```python
from build123d import *

# Parameters (mm, degrees)
SKETCH2_W           = 88.9
SKETCH2_H           = 152.4
BOSS_EXTRUDE1_DEPTH = 10.16
SKETCH5_W           = 57.15
SKETCH5_H           = 50.8
BOSS_EXTRUDE2_DEPTH = 133.35
SKETCH6_R           = 2.5
CUT_EXTRUDE1_DEPTH  = 11.16
SKETCH7_R           = 10.5
CUT_EXTRUDE2_DEPTH  = 58.15
SKETCH8_R           = 16.5
CUT_EXTRUDE3_DEPTH  = 54.15
SKETCH9_R           = 19.5
CUT_EXTRUDE4_DEPTH  = 16.51
BOSS_EXTRUDE3_DEPTH = 3
SKETCH12_R          = 9.525
CUT_EXTRUDE6_DEPTH  = 12.7


with BuildPart() as part:
    # Sketch2 → Boss-Extrude1 (new body)
    with BuildSketch(Plane(origin=(0, 0, 0), x_dir=(1, 0, 0), z_dir=(0, 1, 0))):
        with Locations((8.89, -19.614444444)):
            Rectangle(SKETCH2_W, SKETCH2_H)
    extrude(amount=BOSS_EXTRUDE1_DEPTH)

    # Sketch5 → Boss-Extrude2 (add)
    with BuildSketch(Plane(origin=(0, 10.16, 0), x_dir=(1, 0, 0), z_dir=(0, 1, 0))):
        with Locations((-6.985, -19.614444444)):
            Rectangle(SKETCH5_W, SKETCH5_H)
    extrude(amount=BOSS_EXTRUDE2_DEPTH)

    # Sketch6 → Cut-Extrude1 (cut, through all)
    with BuildSketch(Plane(origin=(0, 10.16, 0), x_dir=(1, 0, 0), z_dir=(0, 1, 0))):
        with Locations((35.84, -88.314444444)):
            Circle(SKETCH6_R)
        with Locations((45.84, -88.314444444)):
            Circle(SKETCH6_R)
        with Locations((-28.06, -88.314444444)):
            Circle(SKETCH6_R)
        with Locations((-18.06, -88.314444444)):
            Circle(SKETCH6_R)
        with Locations((-28.06, 49.085555556)):
            Circle(SKETCH6_R)
        with Locations((-18.06, 49.085555556)):
            Circle(SKETCH6_R)
        with Locations((35.84, 49.085555556)):
            Circle(SKETCH6_R)
        with Locations((45.84, 49.085555556)):
            Circle(SKETCH6_R)
    extrude(amount=-CUT_EXTRUDE1_DEPTH, mode=Mode.SUBTRACT)

    # Sketch7 → Cut-Extrude2 (cut, through all)
    with BuildSketch(Plane(origin=(21.59, 0, 0), x_dir=(0, 0, -1), z_dir=(1, 0, 0))):
        with Locations((-19.614444444, 119.38)):
            Circle(SKETCH7_R)
    extrude(amount=-CUT_EXTRUDE2_DEPTH, mode=Mode.SUBTRACT)

    # Sketch8 → Cut-Extrude3 (cut)
    with BuildSketch(Plane.ZY.offset(35.56)):
        with Locations((19.614444444, 119.38)):
            Circle(SKETCH8_R)
    extrude(amount=-CUT_EXTRUDE3_DEPTH, mode=Mode.SUBTRACT)

    # Sketch9 → Cut-Extrude4 (cut)
    with BuildSketch(Plane.ZY.offset(35.56)):
        with Locations((19.614444444, 119.38)):
            Circle(SKETCH9_R)
    extrude(amount=-CUT_EXTRUDE4_DEPTH, mode=Mode.SUBTRACT)

    # Sketch10 → Boss-Extrude3 (add)
    with BuildSketch(Plane(origin=(21.59, 0, 0), x_dir=(0, 0, -1), z_dir=(1, 0, 0))):
        with BuildLine():
            Line((-29.348407204, 123.317), (-29.348407204, 115.443))
            ThreePointArc((-29.348407204, 115.443), (-30.114444444, 119.38), (-29.348407204, 123.317))
        make_face()
        with BuildLine():
            Line((-9.880481685, 115.443), (-9.880481685, 123.317))
            ThreePointArc((-9.880481685, 123.317), (-9.114444444, 119.38), (-9.880481685, 115.443))
        make_face()
    extrude(amount=-BOSS_EXTRUDE3_DEPTH)

    # Sketch12 → Cut-Extrude6 (cut)
    with BuildSketch(Plane(origin=(0, 10.16, 0), x_dir=(1, 0, 0), z_dir=(0, 1, 0))):
        with Locations((53.34, -70.414444444)):
            Circle(SKETCH12_R)
        with Locations((53.34, 31.185555556)):
            Circle(SKETCH12_R)
    extrude(amount=-CUT_EXTRUDE6_DEPTH, mode=Mode.SUBTRACT)


solid = part.part
```
The listing builds one solid part. Answer for the finished solid, in the listing's coordinates (mm). A direction names the side the tool comes from. Give positions to 0.01 mm unless a question says otherwise; leave off trailing zeros. Loops run counter-clockwise (first coordinate to the right, second up) from the corner with the lowest first, then second, coordinate; pieces in that order, holes last. Notation, with made-up numbers: (64, -27.5) - (112, -27.5) arc R16 ccw to (112, -10.5) - close; hole circle Ø5 at (51, 37.5). An arc over 180 degrees is marked (long way). Return JSON: item names as keys, results as strings. Group by question number.
1. Which of the six approach directions +Z, -Z, +X, -X, +Y, -Y give full straight-line access (tool end or side, diameter ignored) to faces 4 (the cylindrical face through (-27.42, 102.08, 28.61)), 5 (the cylindrical face through (-18.385, 5.151, 85.836)), 6 (the cylindrical face through (20.11, 108.88, 19.79)), 7 (the flat face through (-7, 76, 45.014)), 8 (the flat face through (21.59, 78, 19))?
2. Find section A-A (x = -28.06). Write down the section's boundary in (y, z).
3. Straight lines are drawn through the part: line 1 (Z direction, x = -18, y = 7); line 2 (Z direction, x = 45.84, y = 3); line 3 (Y direction, x = 39, z = 10). For each, find the intervals that lie inside material, in ascending order. Write a range as [from, to].
4. Find section B-B (y = 119.38). Write down the section's boundary in (x, z), then the cut area to 3 significant figures.
5. Determine the mould class of faces 1 (the cylindrical face through (-28.385, 5.151, -51.564)), 2 (the cylindrical face through (-0.49, 135.74, 17.47)), 3 (the flat face through (8, 0, 19)) for opening direction Y: pulls with the +Y half, pulls with the -Y half, needs draft (parallel to the pull), parting line crosses it, or undercut.
6. Find section C-C (x = 4.5). Write down the section's boundary in (y, z), then the cut area to 3 significant figures.
7. Given pin 1 Ø3 at (x, z) = (18, 51) entering from +Y; pin 2 Ø10 at (y, z) = (116.5, 25.5) entering from -X; pin 3 Ø15 at (y, z) = (105, 23) entering from +X, each flat-ended and moving along its own axis, determine where each tip first touches the part or whether it passes through.
8. Find section D-D (x = 45.84). Write down the section's boundary in (y, z), then the cut area to 3 significant figures.
Verdict:
{
 "1": {"face 4": "-X", "face 5": "+Y, -Y", "face 6": "+X, -X", "face 7": "+Z, +X, -X, +Y", "face 8": "+Z, -Z, +X, +Y"},
 "2": {"outline": "(0, -56.59) - (10.16, -56.59) - (10.16, -51.59) - (0, -51.59) - close; (0, -46.59) - (10.16, -46.59) - (10.16, -5.79) - (143.51, -5.79) - (143.51, 45.01) - (10.16, 45.01) - (10.16, 85.81) - (0, 85.81) - close; (0, 90.81) - (10.16, 90.81) - (10.16, 95.81) - (0, 95.81) - close; hole circle Ø39 at (119.38, 19.61)"},
 "3": {"line 1": "z = [-56.59, -51.58], [-46.59, 85.82], [90.81, 95.81]", "line 2": "z = [-56.59, -51.59], [-46.59, -37.06], [-25.31, 64.54], [76.29, 85.81], [90.81, 95.81]", "line 3": "y = [0, 10.16]"},
 "4": {"outline": "(-35.56, -5.79) - (21.59, -5.79) - (21.59, 9.88) - (18.59, 9.88) - (18.59, 3.11) - (-19.05, 3.11) - (-19.05, 0.11) - (-35.56, 0.11) - close; (-35.56, 39.11) - (-19.05, 39.11) - (-19.05, 36.11) - (18.59, 36.11) - (18.59, 29.35) - (21.59, 29.35) - (21.59, 45.01) - (-35.56, 45.01) - close", "area": "959 mm^2"},
 "5": {"face 1": "needs draft", "face 2": "undercut", "face 3": "pulls with the -Y half"},
 "6": {"outline": "(0, -56.59) - (10.16, -56.59) - (10.16, -5.79) - (143.51, -5.79) - (143.51, 45.01) - (10.16, 45.01) - (10.16, 95.81) - (0, 95.81) - close; hole circle Ø33 at (119.38, 19.61)", "area": "7,470 mm^2"},
 "7": {"pin 1": "stops at y = 10.16", "pin 2": "stops at x = 18.59", "pin 3": "stops at x = 21.59"},
 "8": {"outline": "(0, -56.59) - (10.16, -56.59) - (10.16, -51.59) - (0, -51.59) - close; (0, -46.59) - (10.16, -46.59) - (10.16, -37.06) - (0, -37.06) - close; (0, -25.31) - (10.16, -25.31) - (10.16, 64.54) - (0, 64.54) - close; (0, 76.29) - (10.16, 76.29) - (10.16, 85.81) - (0, 85.81) - close; (0, 90.81) - (10.16, 90.81) - (10.16, 95.81) - (0, 95.81) - close", "area": "1,210 mm^2"}
}
